Input: part model. Units: mm. Frame: model coordinates. Face numbers are marked on the shaded views. A direction names the side the tool comes from. Round coordinates to 2 decimals unless told otherwise and drop trailing zeros. Order: outer loops, then holes, each group sorted by start corner. A loop starts at its lowest first (then second) coordinate and runs counter-clockwise, first axis right, second up. Notation, with made-up numbers: M 84,18 L 138,18 A18 ccw 138,36 Z; hole C -25,-26.5 d11. An arc over 180 degrees is marked long. One line per question, with ' | ' between items.
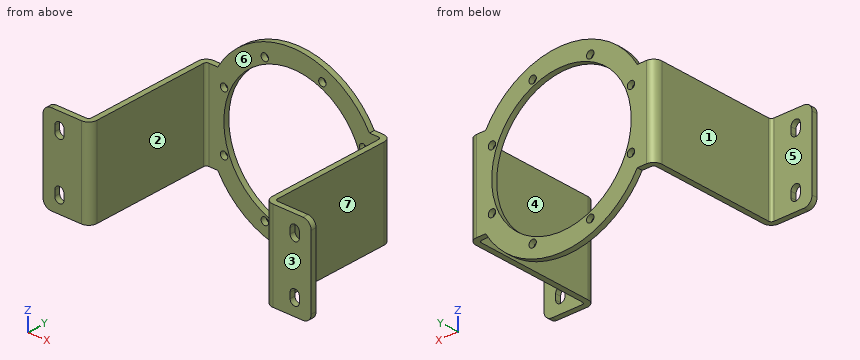
```python
from build123d import *

# Parameters (mm, degrees)
SKETCH_1_R          = 25.5
EXTRUDE_1_DEPTH     = 2
SKETCH_2_W          = 2
SKETCH_2_H          = 32
EXTRUDE_2_DEPTH     = 47.2
SKETCH_3_W          = 32
SKETCH_3_H          = 2
EXTRUDE_3_DEPTH     = 15
FILLET_1_R          = 3
FILLET_2_R          = 1
SKETCH_4_R          = 1.35
CUT_EXTRUDE_1_DEPTH = 10
CUT_EXTRUDE_2_DEPTH = 10
FILLET_3_R          = 3


with BuildPart() as part:
    # 草图1 → 凸台-拉伸1 (new body)
    with BuildSketch(Plane(origin=(0, 53.2, 0), x_dir=(1, 0, 0), z_dir=(0, 1, 0))):
        with BuildLine():
            Line((-34, 16), (-34, -16))
            Line((-34, -16), (-27.712812921, -16))
            ThreePointArc((-27.712812921, -16), (0, -32), (27.712812921, -16))
            Line((27.712812921, -16), (34, -16))
            Line((34, -16), (34, 16))
            Line((34, 16), (27.712812921, 16))
            ThreePointArc((27.712812921, 16), (0, 32), (-27.712812921, 16))
            Line((-27.712812921, 16), (-34, 16))
        make_face()
        with Locations(Location((0, 0, 0), (0, 0, 180))):
            Circle(SKETCH_1_R, mode=Mode.SUBTRACT)
    extrude(amount=EXTRUDE_1_DEPTH)

    # 草图2 → 凸台-拉伸2 (add)
    with BuildSketch(Plane.XZ.offset(-53.2)):
        with Locations((-33, 0)):
            Rectangle(SKETCH_2_W, SKETCH_2_H)
        with Locations((33, 0)):
            Rectangle(SKETCH_2_W, SKETCH_2_H)
    extrude(amount=EXTRUDE_2_DEPTH)

    # 草图3 → 凸台-拉伸3 (add)
    with BuildSketch(Plane.ZY.offset(34)):
        with Locations((0, 7)):
            Rectangle(SKETCH_3_W, SKETCH_3_H)
    extrude_3 = extrude(amount=EXTRUDE_3_DEPTH)

    # 镜向1: 凸台-拉伸3 across plane
    add(extrude_3.mirror(Plane.ZY))

    # 圆角1
    fillet_1_edges = [part.edges().sort_by_distance(p)[0] for p in [
        (34, 55.2, 0),
        (-32, 6, 0),
        (32, 6, 0),
        (-34, 55.2, 0),
    ]]
    fillet(fillet_1_edges, radius=FILLET_1_R)

    # 圆角2
    fillet_2_edges = [part.edges().sort_by_distance(p)[0] for p in [
        (-32, 53.2, 0),
        (32, 53.2, 0),
        (-34, 8, 0),
        (34, 8, 0),
    ]]
    fillet(fillet_2_edges, radius=FILLET_2_R)

    # 草图4 → 切除-拉伸1 (cut)
    with BuildSketch(Plane(origin=(0, 55.2, 0), x_dir=(1, 0, 0), z_dir=(0, 1, 0))):
        with Locations(Location((-10.52379439, 25.406687144, 0), (0, 0, 180))):
            Circle(SKETCH_4_R)
        with Locations(Location((10.52379439, 25.406687144, 0), (0, 0, 180))):
            Circle(SKETCH_4_R)
        with Locations(Location((25.406687144, 10.52379439, 0), (0, 0, 180))):
            Circle(SKETCH_4_R)
        with Locations(Location((25.406687144, -10.52379439, 0), (0, 0, 180))):
            Circle(SKETCH_4_R)
        with Locations(Location((10.52379439, -25.406687144, 0), (0, 0, 180))):
            Circle(SKETCH_4_R)
        with Locations(Location((-10.52379439, -25.406687144, 0), (0, 0, 180))):
            Circle(SKETCH_4_R)
        with Locations(Location((-25.406687144, -10.52379439, 0), (0, 0, 180))):
            Circle(SKETCH_4_R)
        with Locations(Location((-25.406687144, 10.52379439, 0), (0, 0, 180))):
            Circle(SKETCH_4_R)
    extrude(amount=-CUT_EXTRUDE_1_DEPTH, mode=Mode.SUBTRACT)

    # 草图6 → 切除-拉伸2 (cut)
    with BuildSketch(Plane(origin=(0, 8, 0), x_dir=(1, 0, 0), z_dir=(0, 1, 0))):
        with BuildLine():
            Line((-41.3, 11), (-41.3, 9))
            ThreePointArc((-41.3, 9), (-43, 7.3), (-44.7, 9))
            Line((-44.7, 9), (-44.7, 11))
            ThreePointArc((-44.7, 11), (-43, 12.7), (-41.3, 11))
        make_face()
        with BuildLine():
            Line((-41.3, -11), (-41.3, -9))
            ThreePointArc((-41.3, -9), (-43, -7.3), (-44.7, -9))
            Line((-44.7, -9), (-44.7, -11))
            ThreePointArc((-44.7, -11), (-43, -12.7), (-41.3, -11))
        make_face()
    cut_extrude_2 = extrude(amount=-CUT_EXTRUDE_2_DEPTH, mode=Mode.SUBTRACT)

    # 镜向2: 切除-拉伸2 across plane
    add(cut_extrude_2.mirror(Plane.ZY), mode=Mode.SUBTRACT)

    # 圆角3
    fillet_3_edges = [part.edges().sort_by_distance(p)[0] for p in [
        (-49, 7, 16),
        (-49, 7, -16),
        (49, 7, 16),
        (49, 7, -16),
    ]]
    fillet(fillet_3_edges, radius=FILLET_3_R)


solid = part.part
```
Item 1: Section query B-B, the plane z = 0. Return loops of the section in (x, y), plus the area to 3 significant figures.
Report:
outline: M -49,6 L -35,6 A3 ccw -32,9 L -32,52.2 A1 cw -31,53.2 L -25.5,53.2 L -25.5,55.2 L -31,55.2 A3 ccw -34,52.2 L -34,9 A1 cw -35,8 L -49,8 Z; M 25.5,53.2 L 31,53.2 A1 cw 32,52.2 L 32,9 A3 ccw 35,6 L 49,6 L 49,8 L 35,8 A1 cw 34,9 L 34,52.2 A3 ccw 31,55.2 L 25.5,55.2 Z | area: 276 mm²
Item 2: Mould query, pull axis X, two halves, no side actions, for the marked faces 1, 2, 3 and 4. Classes: +X half, -X half, draft (parallel to the pull), parting line (faces both ways), or undercut.
Report:
face 1: -X half | face 2: undercut | face 3: draft | face 4: undercut
Item 3: Section query A-A, the plane y = 46. Return loops of the section in (x, z).
Report:
outline: M -34,-16 L -32,-16 L -32,16 L -34,16 Z; M 32,-16 L 34,-16 L 34,16 L 32,16 Z
Item 4: Section query C-C, the plane x = -43. Return loops of the section in (y, z), plus the area to 3 significant figures.
Report:
outline: M 6,-16 L 8,-16 L 8,-12.7 L 6,-12.7 Z; M 6,-7.3 L 8,-7.3 L 8,7.3 L 6,7.3 Z; M 6,12.7 L 8,12.7 L 8,16 L 6,16 Z | area: 42.4 mm²
Item 5: Line query: line 1 along X through (y, z) = (27.5, 6); line 2 along Y through (x, z) = (-11.5, -23); line 3 along Y through (x, z) = (-36, -9). Output: solid intervals per line, ascending. Write a range as from..to.
Report:
line 1: -34..-32, 32..34 | line 2: 53.2..55.2 | line 3: 6..8
Item 6: First-contact query: pin 1 (5 mm diameter, centred on y = 34.5, z = 9.5, fed in from +X); pin 2 (9.5 mm diameter, centred on y = 25, z = -6, fed in from -X); pin 3 (14.5 mm diameter, centred on x = -38, y = 21.5, fed in from -Z). Flat tips, straight axial feed; report the tip coordinate or a pass-through.
Report:
pin 1: x = 34 | pin 2: x = -34 | pin 3: z = -16
Item 7: Access query for the marked faces 5, 6 and 7. Directions: +Z, -Z, +X, -X, +Y, -Y. A direction counts if a zero-diameter tool reaches every point of the face in a straight line with its end or side. Return the directions, or none.
Report:
face 5: +Z, -Z, -X, +Y | face 6: +Z, -Z, -Y | face 7: +Z, -Z, +X, +Y
